Verification items for this drawing (mm, ordinates from the low corner). Coordinates: 2 decimals unless noted, no trailing zeros. Order: outer loops, then holes, each group sorted by start corner. A loop starts at its lowest first (then second) coordinate and runs counter-clockwise, first axis right, second up. Notation, with made-up numbers: M -38,64 L -6,64 A13 cw -6,71 Z; hole C 65,19 d6. An arc over 180 degrees is marked long. Write item = value, one per line.
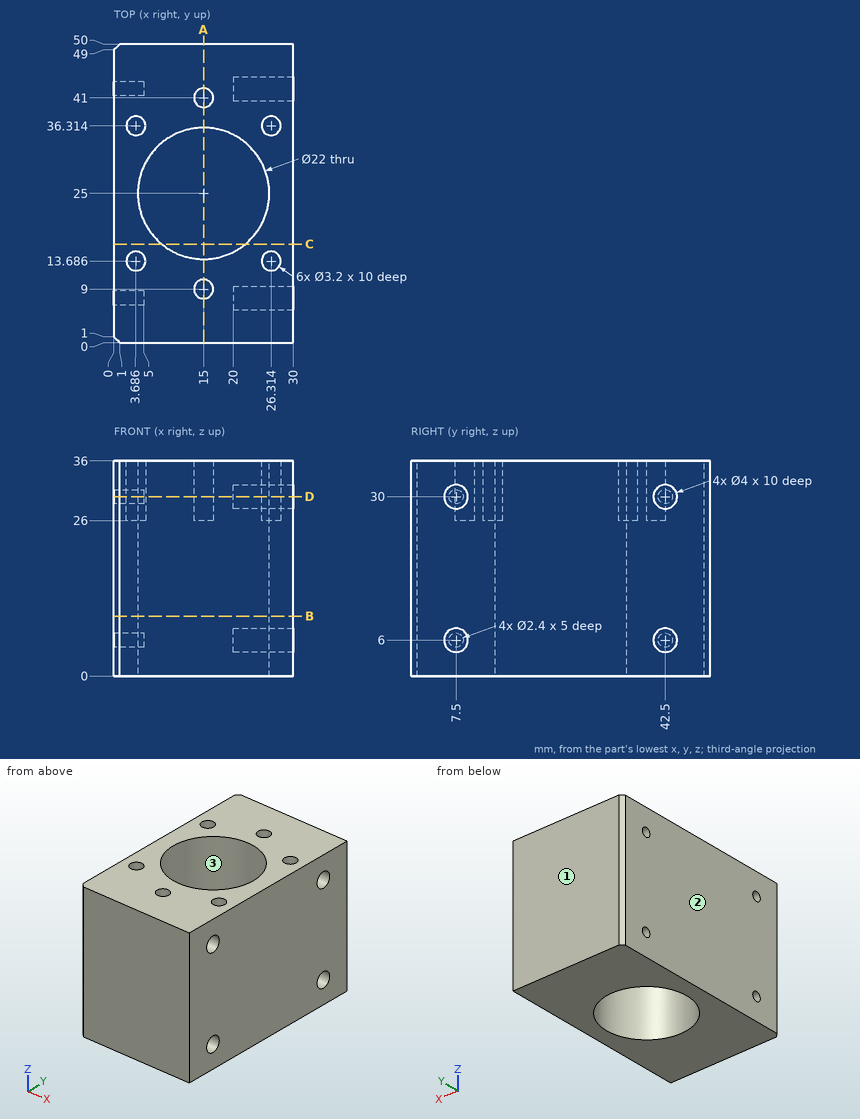
Item 1: Sectioned sample at D-D, the plane z = 30. Give the number of separate pieces and of enclosed holes in the cut face.
Report:
separate_pieces = 1
enclosed_holes = 7
Item 2: Sectioned sample at B-B, the plane z = 10. Enter the section's corners in (x, y), then the cut area to 3 significant figures.
Report:
outline = M 0,1 L 1,0 L 30,0 L 30,50 L 1,50 L 0,49 Z; hole C 15,25 d22
area = 1,120 mm^2
Item 3: Release check for a two-part mould opening along Y. For the marked faces 1, 2 and 3 record: pulls with the +Y half, pulls with the -Y half, needs draft (parallel to the pull), parting line crosses it, or undercut.
Report:
face_1 = pulls with the +Y half
face_2 = needs draft
face_3 = undercut
Item 4: Sectioned sample at A-A, the plane x = 15. Enter the section's corners in (y, z).
Report:
outline = M 0,0 L 14,0 L 14,36 L 10.6,36 L 10.6,26 L 7.4,26 L 7.4,36 L 0,36 Z; M 36,0 L 50,0 L 50,36 L 42.6,36 L 42.6,26 L 39.4,26 L 39.4,36 L 36,36 Z
Item 5: Gauge pin test, flat ends, axial feed: pin 1 (1.2 mm diameter, centred on y = 42.5, z = 30, fed in from -X); pin 2 (1.6 mm diameter, centred on x = 15, y = 41.5, fed in from +Z). Record the tip position at first contact, or that the pin passes through.
Report:
pin_1 = 5
pin_2 = 26
Item 6: Scan lines: L1, parallel to Y at x = 3.6, z = 30; L2, parallel to Y at x = 15, z = 33; L3, parallel to Z at x = 27.75, y = 43. Record each from-to range of solid material in increasing order. Write a range as from..to.
Report:
L1 = 0..6.3, 8.7..12.09, 15.28..34.72, 37.91..41.3, 43.7..50
L2 = 0..7.4, 10.6..14, 36..39.4, 42.6..50
L3 = 0..4.06, 7.94..28.06, 31.94..36
Item 7: Sectioned sample at C-C, the plane y = 16.5. Enter the section's corners in (x, z), then the cut area to 3 significant figures.
Report:
outline = M 0,0 L 8.02,0 L 8.02,36 L 0,36 Z; M 21.98,0 L 30,0 L 30,36 L 21.98,36 Z
area = 577 mm^2
